from build123d import *

# Parameters (mm, degrees)
F0_W     = 63.5
F0_H     = 38.1
F1_DEPTH = 5.08
F2_W     = 50.8
F2_H     = 38.1
F3_DEPTH = 20.32
F4_W     = 40.64
F4_H     = 8.89
F5_DEPTH = 20.32
F7_DEPTH = 50.8


with BuildPart() as f1:
    # F0 (on Front) → F1 (new body)
    with BuildSketch(Plane.XZ):
        with Locations((0.112484, 0.318908)):
            Rectangle(F0_W, F0_H)
    extrude(amount=F1_DEPTH)

    # F2 (on face) → F3 (join)
    with BuildSketch(Plane(origin=(0, 0, 0), x_dir=(-1, 0, 0), z_dir=(0, 1, 0))):
        with Locations((0.2931, 0.318908)):
            Rectangle(F2_W, F2_H)
    extrude(amount=F3_DEPTH)

    # F4 (on face) → F5 (cut)
    with BuildSketch(Plane(origin=(0, 20.32, 0), x_dir=(-1, 0, 0), z_dir=(0, 1, 0))):
        with Locations((0.2931, -14.286092)):
            Rectangle(F4_W, F4_H)
    extrude(amount=-F5_DEPTH, mode=Mode.SUBTRACT)

    # F6 (on face) → F7 (cut)
    with BuildSketch(Plane(origin=(0, 20.32, 0), x_dir=(-1, 0, 0), z_dir=(0, 1, 0))):
        with BuildLine():
            Line((10.4531, 19.368908), (-9.8669, 19.368908))
            ThreePointArc((-9.8669, 19.368908), (0.2931, 9.939267), (10.4531, 19.368908))
        make_face()
    extrude(amount=-F7_DEPTH, mode=Mode.SUBTRACT)


solid = f1.part
Geometry: final body of the model. Coordinates: model frame, mm. A direction names the side the tool comes from. Round coordinates to 2 decimals unless told otherwise and drop trailing zeros. Order: outer loops, then holes, each group sorted by start corner. A loop starts at its lowest first (then second) coordinate and runs counter-clockwise, first axis right, second up. Notation, with made-up numbers: (-26.75, 51) -> (-5.75, 51) arc R20 ccw to (-5.75, 88) -> close; hole circle Ø6 at (4, -34). An arc over 180 degrees is marked (long way). Put each result on its own line as item: value. Start each with the question number.
Q1. Section A-A on z = -16. Return the cut outline in (x, y), and give its area (3 significant figures).
Q2. Pull-direction query (X, two-part tool) for faces 1 (the flat face through (0, 10, -9.841)), 2 (the flat face through (-20.613, 10, -14)), 3 (the flat face through (25.107, 10, 0)), 4 (the flat face through (0, -5.08, 1)); classes: +X half, -X half, draft (parallel to the pull), parting line (faces both ways), or undercut.
Q3. Section C-C on x = -17. Return the cut outline in (y, z), and give its area (3 significant figures).
Q4. Section D-D on z = 1. Return the cut outline in (x, y), and give its area (3 significant figures).
Q5. Section B-B on y = 14.75. Return the cut outline in (x, z), and give its area (3 significant figures).
Q6. Line query: probe 1 along X at (y, z) = (18.75, -13.5); probe 2 along Z at (x, y) = (-10.5, 15); probe 3 along Y at (x, z) = (-26, -9.5). Output: solid intervals per line, ascending.
Q7. Reachability of faces 5 (the flat face through (0, 0, -14)), 6 (the flat face through (28, 0, 1)), 7 (the flat face through (-29, 0, 1)) from +Z, -Z, +X, -X, +Y, -Y: full face, straight path, thin tool, end or side. Return the list, or none.
Q8. First-contact query: pin 1 (2 mm diameter, centred on x = 1, y = 8.5, fed in from -Z); pin 2 (2.5 mm diameter, centred on y = 10, z = -15.5, fed in from -X); pin 3 (6.5 mm diameter, centred on x = -28, z = 6, fed in from +Y); pin 4 (12 mm diameter, centred on y = 10, z = 5, fed in from +X). Flat tips, straight axial feed; report the tip coordinate or a pass-through.
Ans:
1. outline: (-31.64, -5.08) -> (31.86, -5.08) -> (31.86, 0) -> (25.11, 0) -> (25.11, 20.32) -> (20.03, 20.32) -> (20.03, 0) -> (-20.61, 0) -> (-20.61, 20.32) -> (-25.69, 20.32) -> (-25.69, 0) -> (-31.64, 0) -> close
1. area: 529 mm2
2. face 1: undercut
2. face 2: undercut
2. face 3: +X half
2. face 4: draft
3. outline: (-5.08, -18.73) -> (0, -18.73) -> (0, -9.84) -> (20.32, -9.84) -> (20.32, 19.37) -> (-5.08, 19.37) -> close
3. area: 787 mm2
4. outline: (-31.64, -5.08) -> (31.86, -5.08) -> (31.86, 0) -> (25.11, 0) -> (25.11, 20.32) -> (-25.69, 20.32) -> (-25.69, 0) -> (-31.64, 0) -> close
4. area: 1,350 mm2
5. outline: (-25.69, -18.73) -> (-20.61, -18.73) -> (-20.61, -9.84) -> (20.03, -9.84) -> (20.03, -18.73) -> (25.11, -18.73) -> (25.11, 19.37) -> (9.87, 19.37) arc R10.19 cw to (-10.45, 19.37) -> (-25.69, 19.37) -> close
5. area: 1,430 mm2
6. probe 1: x = -25.69 to -20.61, 20.03 to 25.11
6. probe 2: z = -9.84 to 19.37
6. probe 3: y = -5.08 to 0
7. face 5: -Z, +Y
7. face 6: +Z, -Z, +X, +Y
7. face 7: +Z, -Z, -X, +Y
8. pin 1: stops at z = -9.84
8. pin 2: stops at x = -25.69
8. pin 3: stops at y = 20.32
8. pin 4: stops at x = 25.11
